from build123d import *

# Parameters (mm, degrees)
SKETCH1_R               = 12.7
BOSS_EXTRUDE1_DEPTH     = 25.4
SKETCH2_R               = 10.4
CUT_EXTRUDE1_DEPTH      = 5.5
CUT_EXTRUDE2_START      = -1
SKETCH3_R               = 11.75
CUT_EXTRUDE2_DEPTH      = 1.8
F_1_4_28_TAPPED_HOLE1_D = 5.4102
SKETCH11_R              = 1
CUT_EXTRUDE3_DEPTH      = 26.4


with BuildPart() as part:
    # Sketch1 → Boss-Extrude1 (new body)
    with BuildSketch(Plane.XY):
        Circle(SKETCH1_R)
    extrude(amount=BOSS_EXTRUDE1_DEPTH)

    # Sketch2 → Cut-Extrude1 (cut)
    with BuildSketch(Plane(origin=(0, 0, 0), x_dir=(-1, 0, 0), z_dir=(0, 0, -1))):
        Circle(SKETCH2_R)
    extrude(amount=-CUT_EXTRUDE1_DEPTH, mode=Mode.SUBTRACT)

    # Sketch3 → Cut-Extrude2 (cut)
    with BuildSketch(Plane(origin=(0, 0, 0), x_dir=(-1, 0, 0), z_dir=(0, 0, -1)).offset(CUT_EXTRUDE2_START)):
        Circle(SKETCH3_R)
    extrude(amount=-CUT_EXTRUDE2_DEPTH, mode=Mode.SUBTRACT)

    # 1/4-28 Tapped Hole1 (through all)
    with Locations(Plane.XY.offset(25.4)):
        with Locations((0, 0)):
            Hole(F_1_4_28_TAPPED_HOLE1_D / 2)

    # Sketch10 → Cut-Revolve1 (revolve, cut)
    with BuildSketch(Plane(origin=(0, 0, 0), x_dir=(1, 0, 0), z_dir=(0, 1, 0))):
        Polygon((0, -25.402256059), (8.654624222, -5.5), (0, -5.5), align=None)
    revolve(axis=Axis((0, 0, 29.736025406), (0, 0, -1)), mode=Mode.SUBTRACT)

    # Sketch11 → Cut-Extrude3 (cut, through all)
    with BuildSketch(Plane.XY.offset(25.4)):
        with Locations((-7.70255, 0)):
            Circle(SKETCH11_R)
        with Locations((7.70255, 0)):
            Circle(SKETCH11_R)
    extrude(amount=-CUT_EXTRUDE3_DEPTH, mode=Mode.SUBTRACT)


solid = part.part
Check sheet for the modelled part. Datum: model origin and axes. Units: mm. A direction names the side the tool comes from. Round coordinates to 2 decimals unless told otherwise and drop trailing zeros. Write each loop counter-clockwise with the first axis right and the second up, starting at its lowest first coordinate (ties: lowest second). Pieces come first, ordered by that corner, then holes. Notation, with made-up numbers: (74, 16) -> (87, 16) arc R34 ccw to (87, 47) -> close; hole circle Ø5 at (48, 20). An arc over 180 degrees is marked (long way). Answer as CSV lines item,"result". Start each with the question number.
1) Section check A-A on x = 0. Enter the section's corners in (y, z), and give its area (3 significant figures).
2) Section check B-B on z = 21.75. Enter the section's corners in (x, y), and give its area (3 significant figures).
3) Material ranges on line 1 (Y direction, x = 0, z = 1.8); line 2 (Z direction, x = 5.75, y = 9.5); line 3 (Y direction, x = -0.5, z = 7.5), recorded low to high. Write a range as from..to.
4) Tool access check on faces 5 (the flat face through (-10.4, 1.9, 0)), 6 (the flat face through (4, 8, 5.5)), 7 (the cylindrical face through (-11.207, 3.529, 1.887)). Record the directions out of +Z, -Z, +X, -X, +Y, -Y that give a thin tool (end or side, any length) a straight path to the whole face; none if there is none.
5) Section check C-C on z = 13. Enter the section's corners in (x, y), and give its area (3 significant figures).
6) Release check for a two-part mould opening along Z. For faces 1 (the flat face through (-4, -10, 1)), 2 (the flat face through (-4, -10, 2.8)), 3 (the conical face through (4.67, 1.94, 13.77)), 4 (the cylindrical face through (-8.7, 0.04, 15.59)) record: pulls with the +Z half, pulls with the -Z half, needs draft (parallel to the pull), parting line crosses it, or undercut.
7) Go/stop test with flat-tipped pins: P1, Ø1, axis at x = 2.5, z = 17.5, coming from the -Y side; P2, Ø4, axis at y = -2.5, z = 4, coming from the -X side; P3, Ø8, axis at x = 0.5, y = 5.5, coming from the -Z side. Record where each tip stops, or that it passes through.
Found:
1,outline,"(-12.7, 0) -> (-10.4, 0) -> (-10.4, 1) -> (-11.75, 1) -> (-11.75, 2.8) -> (-10.4, 2.8) -> (-10.4, 5.5) -> (-8.65, 5.5) -> (-2.71, 19.18) -> (-2.71, 25.4) -> (-12.7, 25.4) -> close; (2.71, 19.18) -> (8.65, 5.5) -> (10.4, 5.5) -> (10.4, 2.8) -> (11.75, 2.8) -> (11.75, 1) -> (10.4, 1) -> (10.4, 0) -> (12.7, 0) -> (12.7, 25.4) -> (2.71, 25.4) -> close"
1,area,"337 mm^2"
2,outline,"circle Ø25.4 at (0, 0); hole circle Ø2 at (-7.7, 0); hole circle Ø5.41 at (0, 0); hole circle Ø2 at (7.7, 0)"
2,area,"477 mm^2"
3,line 1,"y = -12.7..-11.75, 11.75..12.7"
3,line 2,"z = 0..1, 2.8..25.4"
3,line 3,"y = -12.69..-7.77, 7.77..12.69"
4,face 5,"-Z, +X, -X, +Y, -Y"
4,face 6,"-Z"
4,face 7,"none"
5,outline,"circle Ø25.4 at (0, 0); hole circle Ø2 at (-7.7, 0); hole circle Ø10.79 at (0, 0); hole circle Ø2 at (7.7, 0)"
5,area,"409 mm^2"
6,face 1,"undercut"
6,face 2,"undercut"
6,face 3,"pulls with the -Z half"
6,face 4,"needs draft"
7,P1,"stops at y = -12.54"
7,P2,"stops at x = -12.69"
7,P3,"stops at z = 5.5"
